Could you check a few things on this model? Use its own coordinates, in mm. Round coordinates to 2 decimals unless told otherwise and drop trailing zeros. Loops run counter-clockwise (first coordinate to the right, second up) from the corner with the lowest first, then second, coordinate; pieces in that order, holes last. Notation, with made-up numbers: (82, 37) -> (100, 37) arc R13 cw to (100, 62) -> close; hole circle Ø10 at (31, 3). An arc over 180 degrees is marked (long way). One line per item, written item: value.
```python
from build123d import *

# Parameters (mm, degrees)
F0_R     = 10
F1_DEPTH = 25
F2_SIZE2 = 6.2
F2_SIZE  = 10.7387150069
F3_R     = 3.8
F4_DEPTH = 40.7
F5_R     = 8
F6_DEPTH = 10.2


with BuildPart() as f1:
    # F0 (on Top) → F1 (new body)
    with BuildSketch(Plane.XY):
        Circle(F0_R)
    extrude(amount=F1_DEPTH)

    # F2
    f2_edges = [f1.edges().sort_by_distance(p)[0] for p in [
        (-10, 0, 25),
    ]]
    f2_side = f1.faces().sort_by_distance((-10, 0, 12.5))[0]
    chamfer(f2_edges, length=F2_SIZE, length2=F2_SIZE2, reference=f2_side)

    # F3 (on face) → F4 (cut)
    with BuildSketch(Plane.XY.offset(25)):
        Circle(F3_R)
    extrude(amount=-F4_DEPTH, mode=Mode.SUBTRACT)

    # F5 (on Top) → F6 (cut)
    with BuildSketch(Plane.XY):
        Circle(F5_R)
    extrude(amount=F6_DEPTH, mode=Mode.SUBTRACT)


solid = f1.part
```
(1) We'd pull the mould along X, two halves only. Please class faces 1 (the face through (0, 8.2, 0)), 2 (the face through (5.226, 1.646, 22.092)), 3 (the face through (-1.73, -7.81, 5.03)), 4 (the face through (-4, -2, 10.2)): +X half, -X half, draft (parallel to the pull), parting line (faces both ways), or undercut.
Results below:
face 1: draft
face 2: parting line
face 3: undercut
face 4: undercut
(2) Imagine slicing it at C-C on z = 2.25. Write out the boundary of the cut face in (x, y), then the cut area to 3 significant figures.
Results below:
outline: circle Ø20 at (0, 0); hole circle Ø16 at (0, 0)
area: 113 mm²
(3) Imagine slicing it at D-D on z = 18. Write out the boundary of the cut face in (x, y), then the cut area to 3 significant figures.
Results below:
outline: circle Ø15.68 at (0, 0); hole circle Ø7.6 at (0, 0)
area: 148 mm²
(4) Imagine slicing it at A-A on x = 0. Write out the boundary of the cut face in (y, z).
Results below:
outline: (-10, 0) -> (-8, 0) -> (-8, 10.2) -> (-3.8, 10.2) -> (-3.8, 25) -> (-10, 14.26) -> close; (3.8, 10.2) -> (8, 10.2) -> (8, 0) -> (10, 0) -> (10, 14.26) -> (3.8, 25) -> close
(5) Please list where these lines run through material, in increasing order: L1, parallel to Y at x = 0, z = 14; L2, parallel to Y at x = 0, z = 4; L3, parallel to X at y = 2.75, z = 2.75.
Results below:
L1: y = -10 to -3.8, 3.8 to 10
L2: y = -10 to -8, 8 to 10
L3: x = -9.61 to -7.51, 7.51 to 9.61
(6) For pin 1 Ø3 at (x, y) = (-3.5, -1.5) entering from -Z; pin 2 Ø5 at (x, z) = (3, 9.5) entering from +Y; pin 3 Ø8 at (y, z) = (7.5, 12.5) entering from -X, each with a flat end and sliding along its axis, tell me the tip position at first contact or that it passes through.
Results below:
pin 1: stops at z = 10.2
pin 2: stops at y = 9.99
pin 3: stops at x = -9.37
